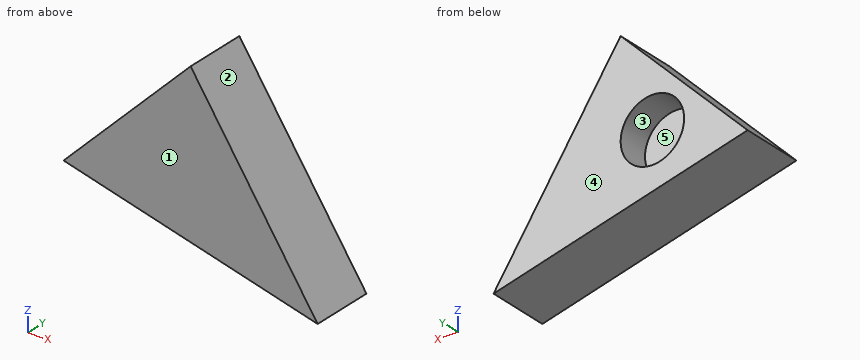
```python
from build123d import *

# Parameters (mm, degrees)
BOSS_EXTRUDE1_DEPTH = 25.4
SKETCH2_R           = 12.7
CUT_EXTRUDE1_DEPTH  = 12.7


with BuildPart() as part:
    # Sketch1 → Boss-Extrude1 (new body)
    with BuildSketch(Plane(origin=(0, 0, 0), x_dir=(1, 0, 0), z_dir=(0, 1, 0))):
        Polygon((0, 0), (50.8, -50.8), (101.6, 25.4), align=None)
    extrude(amount=BOSS_EXTRUDE1_DEPTH)

    # Sketch2 → Cut-Extrude1 (cut)
    with BuildSketch(Plane(origin=(0, 25.4, 0), x_dir=(1, 0, 0), z_dir=(0, 1, 0))):
        with Locations((38.1, -12.7)):
            Circle(SKETCH2_R)
    extrude(amount=-CUT_EXTRUDE1_DEPTH, mode=Mode.SUBTRACT)


solid = part.part
```
For this review, take the finished solid that the model builds, in its own axes (mm). Face numbers are marked on the shaded views. A direction names the side the tool comes from. Give positions to 0.01 mm unless a question says otherwise; leave off trailing zeros. Write each loop counter-clockwise with the first axis right and the second up, starting at its lowest first coordinate (ties: lowest second). Pieces come first, ordered by that corner, then holes. Notation, with made-up numbers: M 52,-13.5 L 75,-13.5 A19 ccw 75,18.5 Z; hole C -7,15 d10. An arc over 180 degrees is marked long. Answer as a JSON object with one key per item and string values. Group by question number.
Item 1: Consider section A-A on z = 12.7. Write out the cut boundary in (x, y), plus the area to 3 significant figures.
Item 2: Consider section C-C on x = 40.5. Write out the cut boundary in (y, z) (3 decimals).
Item 3: For probe 1 along X at (y, z) = (17, 21.5); probe 2 along X at (y, z) = (20, 9.5); probe 3 along Z at (x, y) = (38.1, 20.75) (3 decimals), list the stretches that pass through material, from the lowest coordinate up. Write a range as [from, to].
Item 4: Consider section B-B on y = 19.25. Write out the cut boundary in (x, z).
Item 5: Tool access review of the marked faces 4 and 5: name each direction out of +Z, -Z, +X, -X, +Y, -Y from which nothing blocks a thin tool from reaching the whole face with its end or side.
Item 6: Consider section D-D on y = 3.25. Write out the cut boundary in (x, z), plus the area to 3 significant figures.
Item 7: Draft analysis for pull direction X (two halves, no side actions). For the marked faces 1, 2 and 3, state which applies: +X half, -X half, draft (parallel to the pull), parting line (faces both ways), or undercut.
Item 8: For pin 1 Ø4 at (y, z) = (11, 42) entering from -X; pin 2 Ø6 at (x, z) = (34.5, 11) entering from +Y; pin 3 Ø8 at (y, z) = (20, -16) entering from +X, all flat-tipped, find the tip position at first contact; note any pin that passes through.
Check result:
{
 "1": {"outline": "M 12.7,0 L 76.2,0 L 76.2,25.4 L 50.8,25.4 L 50.8,12.7 L 25.4,12.7 L 25.4,25.4 L 12.7,25.4 Z", "area": "1,290 mm^2"},
 "2": {"outline": "M 0,-10.125 L 25.4,-10.125 L 25.4,0.229 L 12.7,0.229 L 12.7,25.171 L 25.4,25.171 L 25.4,40.5 L 0,40.5 Z"},
 "3": {"probe 1": "x = [21.5, 28.94], [47.26, 70.33]", "probe 2": "x = [9.5, 25.81], [50.39, 78.33]", "probe 3": "z = [-9.525, 0], [25.4, 38.1]"},
 "4": {"outline": "M 0,0 L 101.6,-25.4 L 50.8,50.8 Z; hole C 38.1,12.7 d25.4"},
 "5": {"face 4": "+Z, -Z, +X, -X, +Y", "face 5": "+Y"},
 "6": {"outline": "M 0,0 L 101.6,-25.4 L 50.8,50.8 Z", "area": "3,230 mm^2"},
 "7": {"face 1": "draft", "face 2": "+X half", "face 3": "undercut"},
 "8": {"pin 1": "stops at x = 40", "pin 2": "stops at y = 12.7", "pin 3": "stops at x = 98"}
}
